For this review, take the finished solid that the model builds, in its own axes (mm). Face numbers are marked on the shaded views. A direction names the side the tool comes from. Give positions to 0.01 mm unless a question says otherwise; leave off trailing zeros. Write each loop counter-clockwise with the first axis right and the second up, starting at its lowest first coordinate (ties: lowest second). Pieces come first, ordered by that corner, then holes. Notation, with made-up numbers: (-27, 80) -> (-12, 80) arc R22 ccw to (-12, 93) -> close; hole circle Ø1 at (52.25, 40). An arc over 180 degrees is marked (long way). Return JSON: item names as keys, results as strings.
from build123d import *

# Parameters (mm, degrees)
F0_W     = 95.25
F0_H     = 25.4
F1_DEPTH = 76.2
F2_R     = 7.35111
F2_R_2   = 6.900606
F3_DEPTH = 7.1374
F4_R     = 23.749
F5_DEPTH = 35.1103


with BuildPart() as f1:
    # F0 (on Top) → F1 (new body)
    with BuildSketch(Plane.XY):
        with Locations((-1.087826, 2.483681)):
            Rectangle(F0_W, F0_H)
    extrude(amount=F1_DEPTH)

    # F2 (on face) → F3 (cut)
    with BuildSketch(Plane.XY.offset(76.2)):
        with Locations((36.106295, 2.483681)):
            Circle(F2_R)
        with Locations((-40.093705, 2.483681)):
            Circle(F2_R_2)
    extrude(amount=-F3_DEPTH, mode=Mode.SUBTRACT)

    # F4 (on face) → F5 (cut)
    with BuildSketch(Plane.XZ.offset(10.216319)):
        with Locations((-1.214826, 38.1)):
            Circle(F4_R)
    extrude(amount=-F5_DEPTH, mode=Mode.SUBTRACT)


solid = f1.part
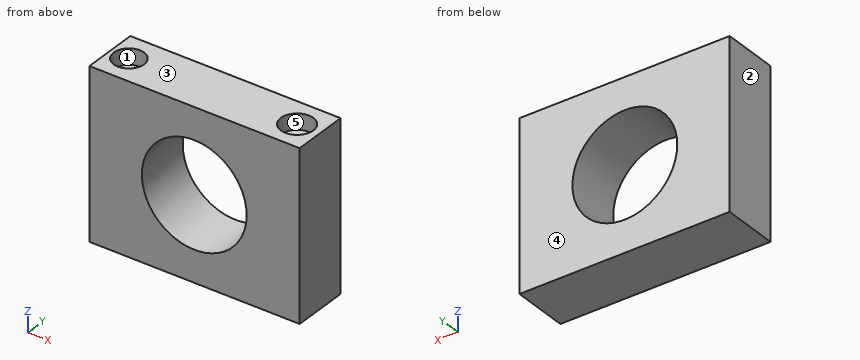
1. Add section C-C, the plane y = 13. State the section outline as (x, z) points, plus the area to 3 significant figures.
Results found:
{"outline": "(-48.71, 0) -> (46.54, 0) -> (46.54, 76.2) -> (-48.71, 76.2) -> close; hole circle Ø47.5 at (-1.21, 38.1)", "area": "5,490 mm²"}
2. Add section B-B, the plane x = 15. State the section outline as (y, z) points, plus the area to 3 significant figures.
Results found:
{"outline": "(-10.22, 0) -> (15.18, 0) -> (15.18, 20.75) -> (-10.22, 20.75) -> close; (-10.22, 55.45) -> (15.18, 55.45) -> (15.18, 76.2) -> (-10.22, 76.2) -> close", "area": "1,050 mm²"}
3. Add section A-A, the plane z = 38.1. State the section outline as (x, y) points, plus the area to 3 significant figures.
Results found:
{"outline": "(-48.71, -10.22) -> (-24.96, -10.22) -> (-24.96, 15.18) -> (-48.71, 15.18) -> close; (22.53, -10.22) -> (46.54, -10.22) -> (46.54, 15.18) -> (22.53, 15.18) -> close", "area": "1,210 mm²"}
4. To check wall thickness, follow probe 1 along X at (y, z) = (3.75, 37.5); probe 2 along X at (y, z) = (9, 49.5); probe 3 along Z at (x, y) = (6, 14.25). State the ranges of each line that lie inside material, in increasing order.
Results found:
{"probe 1": "x = -48.71 to -24.96, 22.53 to 46.54", "probe 2": "x = -48.71 to -22.05, 19.62 to 46.54", "probe 3": "z = 0 to 15.47, 60.73 to 76.2"}
5. For the marked faces 1 and 2, list the 3-axis set-ups (+Z, -Z, +X, -X, +Y, -Y) from which the entire face can be reached by the end or side of a thin tool; tool diameter is ignored.
Results found:
{"face 1": "+Z", "face 2": "+Z, -Z, -X, +Y, -Y"}
6. For pin 1 (10 mm diameter, centred on x = -9, y = 12, fed in from -Z); pin 2 (4.5 mm diameter, centred on x = 39.5, y = 4, fed in from +Z), all flat-tipped, find the tip position at first contact; note any pin that passes through.
Results found:
{"pin 1": "stops at z = 0", "pin 2": "stops at z = 69.06"}
7. The part is to be moulded in two halves that separate along Y. For the marked faces 3, 4 and 5, say which applies: +Y half, -Y half, draft (parallel to the pull), parting line (faces both ways), or undercut.
Results found:
{"face 3": "draft", "face 4": "+Y half", "face 5": "undercut"}
8. Add section D-D, the plane x = 36. State the section outline as (y, z) points, plus the area to 3 significant figures.
Results found:
{"outline": "(-10.22, 0) -> (15.18, 0) -> (15.18, 76.2) -> (9.83, 76.2) -> (9.83, 69.06) -> (-4.87, 69.06) -> (-4.87, 76.2) -> (-10.22, 76.2) -> close", "area": "1,830 mm²"}
